```python
from build123d import *

# Parameters (mm, degrees)
BOSS_EXTRUDE1_DEPTH = 273
SKETCH3_R           = 1.85
SKETCH3_R_2         = 5
CUT_EXTRUDE1_DEPTH  = 273
SKETCH5_R           = 1.55
CUT_EXTRUDE2_DEPTH  = 220


with BuildPart() as part:
    # Sketch1 → Boss-Extrude1 (new body)
    with BuildSketch(Plane.XY):
        Polygon((14, 6.5), (15.5, 6.5), (15.5, -6.5), (-15.5, -6.5), (-15.5, 6.5), (-14, 6.5), (-14, -5), (14, -5), align=None)
    extrude(amount=BOSS_EXTRUDE1_DEPTH)

    # Sketch3 → Cut-Extrude1 (cut)
    with BuildSketch(Plane(origin=(0, -5, 0), x_dir=(1, 0, 0), z_dir=(0, 1, 0))):
        with Locations(Location((-5.656854249, -4.343145751, 0), (0, 0, 270))):
            Circle(SKETCH3_R)
        with Locations(Location((0, -263, 0), (0, 0, 270))):
            Circle(SKETCH3_R_2)
        with Locations(Location((-5.656854249, -257.343145751, 0), (0, 0, 270))):
            Circle(SKETCH3_R)
        with Locations(Location((5.656854249, -257.343145751, 0), (0, 0, 270))):
            Circle(SKETCH3_R)
        with Locations(Location((5.656854249, -268.656854249, 0), (0, 0, 270))):
            Circle(SKETCH3_R)
        with Locations(Location((-5.656854249, -268.656854249, 0), (0, 0, 270))):
            Circle(SKETCH3_R)
        with Locations(Location((5.656854249, -4.343145751, 0), (0, 0, 270))):
            Circle(SKETCH3_R)
        with Locations(Location((5.656854249, -15.656854249, 0), (0, 0, 270))):
            Circle(SKETCH3_R)
        with Locations(Location((-5.656854249, -15.656854249, 0), (0, 0, 270))):
            Circle(SKETCH3_R)
        with Locations(Location((0, -10, 0), (0, 0, 270))):
            Circle(SKETCH3_R_2)
    extrude(amount=-CUT_EXTRUDE1_DEPTH, mode=Mode.SUBTRACT)

    # Sketch5 → Cut-Extrude2 (cut)
    with BuildSketch(Plane.XZ.offset(6.5)):
        with Locations(Location((-10, 229.5, 0), (0, 0, 270))):
            Circle(SKETCH5_R)
        with Locations(Location((-10, 241.5, 0), (0, 0, 270))):
            Circle(SKETCH5_R)
        with Locations(Location((10, 229.5, 0), (0, 0, 270))):
            Circle(SKETCH5_R)
        with Locations(Location((10, 241.5, 0), (0, 0, 270))):
            Circle(SKETCH5_R)
        with Locations(Location((10, 31.5, 0), (0, 0, 270))):
            Circle(SKETCH5_R)
        with Locations(Location((10, 43.5, 0), (0, 0, 270))):
            Circle(SKETCH5_R)
        with Locations(Location((-10, 31.5, 0), (0, 0, 270))):
            Circle(SKETCH5_R)
        with Locations(Location((-10, 43.5, 0), (0, 0, 270))):
            Circle(SKETCH5_R)
    extrude(amount=-CUT_EXTRUDE2_DEPTH, mode=Mode.SUBTRACT)


solid = part.part
```
Check sheet for the modelled part. Datum: model origin and axes. Units: mm. A direction names the side the tool comes from. Coordinates: 2 decimals unless noted, no trailing zeros. Loops run counter-clockwise (first coordinate to the right, second up) from the corner with the lowest first, then second, coordinate; pieces in that order, holes last.
1) Sectioned sample at A-A (z = 263). Record the boundary of the cut face in (x, y).
2) Gauge pin test, flat ends, axial feed: pin 1 (1.9 mm diameter, centred on x = 10, z = 241.5, fed in from +Y); pin 2 (6 mm diameter, centred on x = 5.66, z = 15.66, fed in from +Y). Record the tip position at first contact, or that the pin passes through.
3) Release check for a two-part mould opening along Z. For faces 3 (the face through (1.5, -5.74, 14.77)), 4 (the face through (0, -6, 273)), 5 (the face through (1.5, -5.74, 267.77)), 6 (the face through (14, 1, 135)) record: released by +Z, released by -Z, zero draft, split by the parting line, or undercut.
4) Access from +Z, -Z, +X, -X, +Y, -Y to the whole of each face (thin tool, end or side, straight path). Record for faces 1 (the face through (15.5, 0, 135)), 2 (the face through (-14, 1, 135)).
5) Sectioned sample at C-C (z = 156.5). Record the boundary of the cut face in (x, y), and give its area (3 significant figures).
6) Sectioned sample at B-B (y = 0.5). Record the boundary of the cut face in (x, z), and give its area (3 significant figures).
7) Material ranges on probe 1 along X at (y, z) = (-5.55, 31.5); probe 2 along X at (y, z) = (-1.25, 138); probe 3 along Y at (x, z) = (-5.5, 37.5), recorded low to high.
Check sheet entries:
1. outline: (-15.5, -6.5) - (-5, -6.5) - (-5, -5) - (-14, -5) - (-14, 6.5) - (-15.5, 6.5) - close; (5, -6.5) - (15.5, -6.5) - (15.5, 6.5) - (14, 6.5) - (14, -5) - (5, -5) - close
2. pin 1: passes through
2. pin 2: stops at y = -5
3. face 3: undercut
3. face 4: released by +Z
3. face 5: undercut
3. face 6: zero draft
4. face 1: +Z, -Z, +X, +Y, -Y
4. face 2: +Z, -Z, +Y
5. outline: (-15.5, -6.5) - (15.5, -6.5) - (15.5, 6.5) - (14, 6.5) - (14, -5) - (-14, -5) - (-14, 6.5) - (-15.5, 6.5) - close
5. area: 81.0 mm2
6. outline: (-15.5, 0) - (-14, 0) - (-14, 273) - (-15.5, 273) - close; (14, 0) - (15.5, 0) - (15.5, 273) - (14, 273) - close
6. area: 819 mm2
7. probe 1: x = -15.5 to -11.55, -8.45 to 8.45, 11.55 to 15.5
7. probe 2: x = -15.5 to -14, 14 to 15.5
7. probe 3: y = -6.5 to -5
